Build history of the part. All positions in model axes, mm. Round coordinates to 2 decimals unless told otherwise and drop trailing zeros. Loops run counter-clockwise (first coordinate to the right, second up) from the corner with the lowest first, then second, coordinate; pieces in that order, holes last. Notation, with made-up numbers: (23.5, 66) - (59.5, 66) arc R30 ccw to (59.5, 100) - close; hole circle Ø2 at (15, 16). An arc over 180 degrees is marked (long way). Use a Markdown table: item, result.
from build123d import *

# Parameters (mm, degrees)
SKETCH1_R           = 12.7
SKETCH1_R_2         = 1.397
BOSS_EXTRUDE1_DEPTH = 3.048


with BuildPart() as part:
    # Sketch1 → Boss-Extrude1 (new body)
    with BuildSketch(Plane(origin=(0, 0, 0), x_dir=(1, 0, 0), z_dir=(0, 1, 0))):
        Polygon((0, 0), (15.875, 0), (15.875, 3.048), (31.75, 3.048), (31.75, 0), (47.625, 0), (47.625, 3.048), (63.5, 3.048), (63.5, 0), (95.25, 0), (95.25, 3.048), (111.125, 3.048), (111.125, 0), (127, 0), (127, 3.048), (142.875, 3.048), (142.875, 0), (158.75, 0), (158.75, 15.875), (155.702, 15.875), (155.702, 31.75), (158.75, 31.75), (158.75, 47.625), (155.702, 47.625), (155.702, 63.5), (158.75, 63.5), (158.75, 95.25), (155.702, 95.25), (155.702, 111.125), (158.75, 111.125), (158.75, 127), (155.702, 127), (155.702, 142.875), (158.75, 142.875), (158.75, 158.75), (142.875, 158.75), (142.875, 155.702), (127, 155.702), (127, 158.75), (111.125, 158.75), (111.125, 155.702), (95.25, 155.702), (95.25, 158.75), (63.5, 158.75), (63.5, 155.702), (47.625, 155.702), (47.625, 158.75), (31.75, 158.75), (31.75, 155.702), (15.875, 155.702), (15.875, 158.75), (0, 158.75), (0, 142.875), (3.048, 142.875), (3.048, 127), (0, 127), (0, 111.125), (3.048, 111.125), (3.048, 95.25), (0, 95.25), (0, 63.5), (3.048, 63.5), (3.048, 47.625), (0, 47.625), (0, 31.75), (3.048, 31.75), (3.048, 15.875), (0, 15.875), align=None)
        with Locations((79.375, 79.375)):
            Circle(SKETCH1_R, mode=Mode.SUBTRACT)
        with Locations((73.025, 153.67)):
            Circle(SKETCH1_R_2, mode=Mode.SUBTRACT)
        with Locations((85.725, 153.67)):
            Circle(SKETCH1_R_2, mode=Mode.SUBTRACT)
        with Locations((153.67, 73.025)):
            Circle(SKETCH1_R_2, mode=Mode.SUBTRACT)
        with Locations((153.67, 85.725)):
            Circle(SKETCH1_R_2, mode=Mode.SUBTRACT)
        with Locations((5.08, 85.725)):
            Circle(SKETCH1_R_2, mode=Mode.SUBTRACT)
        with Locations((5.08, 73.025)):
            Circle(SKETCH1_R_2, mode=Mode.SUBTRACT)
        with Locations((73.025, 5.08)):
            Circle(SKETCH1_R_2, mode=Mode.SUBTRACT)
        with Locations((85.725, 5.08)):
            Circle(SKETCH1_R_2, mode=Mode.SUBTRACT)
    extrude(amount=BOSS_EXTRUDE1_DEPTH)


solid = part.part
Q1. Pull direction X, two halves, no side cores. Call faces 1 (the face through (66.687, 1.503, -79.933)), 2 (the face through (96, 0, -80)): pulls with the +X half, pulls with the -X half, needs draft (parallel to the pull), parting line crosses it, or undercut.
Results found:
| item | result |
|---|---|
| face 1 | undercut |
| face 2 | needs draft |
Q2. Drop flat-ended pins along their axis: pin 1 (1.5 mm diameter, centred on y = 1, z = -107, fed in from +X); pin 2 (0.9 mm diameter, centred on x = 100.5, y = 2, fed in from +Z). Give the stop position or say it passes through.
Results found:
| item | result |
|---|---|
| pin 1 | stops at x = 155.7 |
| pin 2 | stops at z = -3.05 |
Q3. Cut at B-B, the plane z = -100. List the corners of the cut face in (x, y), plus the area to 3 significant figures.
Results found:
| item | result |
|---|---|
| outline | (3.05, 0) - (155.7, 0) - (155.7, 3.05) - (3.05, 3.05) - close |
| area | 465 mm2 |
Q4. Probe line 1 (X direction, y = 1, z = -5.08); line 2 (Z direction, x = 153.67, y = 2.05); line 3 (Z direction, x = 141, y = 2.65). List the from-to ranges inside material, lowest first.
Results found:
| item | result |
|---|---|
| line 1 | x = 0 to 71.63, 74.42 to 84.33, 87.12 to 158.75 |
| line 2 | z = -158.75 to -87.12, -84.33 to -74.42, -71.63 to 0 |
| line 3 | z = -155.7 to -3.05 |
Q5. Cut at A-A, the plane x = 81. List the corners of the cut face in (y, z), plus the area to 3 significant figures.
Results found:
| item | result |
|---|---|
| outline | (0, -158.75) - (3.05, -158.75) - (3.05, -91.97) - (0, -91.97) - close; (0, -66.78) - (3.05, -66.78) - (3.05, 0) - (0, 0) - close |
| area | 407 mm2 |
Q6. Cut at D-D, the plane y = 1.95. Count the separate pieces of the cut face and the enclosed holes in it, plus the area to 3 significant figures.
Results found:
| item | result |
|---|---|
| separate pieces | 1 |
| enclosed holes | 9 |
| area | 23,900 mm2 |
Q7. Cut at C-C, the plane x = 132.5. List the corners of the cut face in (y, z), plus the area to 3 significant figures.
Results found:
| item | result |
|---|---|
| outline | (0, -155.7) - (3.05, -155.7) - (3.05, -3.05) - (0, -3.05) - close |
| area | 465 mm2 |
